from build123d import *

# Parameters (mm, degrees)
F1_DEPTH = 21
F2_R     = 3
F3_R     = 3


with BuildPart() as f1:
    # F0 (on Front) → F1 (new body)
    with BuildSketch(Plane.XZ):
        with BuildLine():
            Line((54.864183, -44.821762), (60.732431, -16.421697))
            ThreePointArc((60.732431, -16.421697), (-0.345751, 0.375658), (-61.26627, -16.984813))
            Line((-61.26627, -16.984813), (-53.135817, -44.821762))
            ThreePointArc((-53.135817, -44.821762), (0.864183, -38.821762), (54.864183, -44.821762))
        make_face()
    extrude(amount=F1_DEPTH)

    # F2
    f2_edges = [f1.edges().sort_by_distance(p)[0] for p in [
        (-0.345751, -21, 0.375658),
    ]]
    fillet(f2_edges, radius=F2_R)

    # F3
    f3_edges = [f1.edges().sort_by_distance(p)[0] for p in [
        (-0.345751, 0, 0.375658),
        (0.864183, -21, -38.821762),
        (0.864183, 0, -38.821762),
    ]]
    fillet(f3_edges, radius=F3_R)


solid = f1.part
Build history of the part. All positions in model axes, mm. Coordinates: 2 decimals unless noted, no trailing zeros. Write each loop counter-clockwise with the first axis right and the second up, starting at its lowest first coordinate (ties: lowest second). Pieces come first, ordered by that corner, then holes. Notation, with made-up numbers: (-0.5, 62) -> (37.5, 62) arc R32 ccw to (37.5, 101) -> close; hole circle Ø4 at (-31, 75). An arc over 180 degrees is marked (long way). Use CSV: the item, a comma, the result in double quotes. Start each with the question number.
Q1. Cut at A-A, the plane y = -14. List the corners of the cut face in (x, z).
Q2. Cut at B-B, the plane z = -32.5. List the corners of the cut face in (x, y).
Q3. Drill centre lines: probe 1 along Z at (x, y) = (14, -4.75); probe 2 along Z at (x, y) = (20.5, -18.25); probe 3 along X at (y, z) = (-4, -35). Where is each one in solid material? Low to high.
Q4. Pull direction X, two halves, no side cores. Call faces 1 (the flat face through (-57.258, -10.353, -30.708)), 2 (the flat face through (-1, 0, -22)), 3 (the cylindrical face through (0.102, -10.395, -38.823)), 4 (the flat face through (57.757, -10.353, -30.821)): released by +X, released by -X, zero draft, split by the parting line, or undercut.
Q5. Flat gauge pins, fed straight in: pin 1 Ø6 at (x, y) = (-12, -9) entering from -Z; pin 2 Ø3 at (x, y) = (-36, -11.5) entering from +Z; pin 3 Ø5 at (y, z) = (-7.5, -34.5) entering from -X. Where does each tip first touch, or does it go through?
Checked values:
1,outline,"(-61.27, -16.98) -> (-53.14, -44.82) arc R246 cw to (54.86, -44.82) -> (60.73, -16.42) arc R117.47 ccw to start"
2,outline,"(-56.73, -21) -> (57.41, -21) -> (57.41, 0) -> (-56.73, 0) -> close"
3,probe 1,"z = -39.17 to -0.44"
3,probe 2,"z = -39.6 to -1.4"
3,probe 3,"x = -56 to 56.89"
4,face 1,"released by -X"
4,face 2,"zero draft"
4,face 3,"undercut"
4,face 4,"released by +X"
5,pin 1,"stops at z = -39.33"
5,pin 2,"stops at z = -4.86"
5,pin 3,"stops at x = -56.88"
